from build123d import *

# Parameters (mm, degrees)
SKETCH1_W                    = 63.5
SKETCH1_H                    = 152.4
BASE_FLANGE1_DEPTH           = 1.5875
EDGE_FLANGE1_STRIP_W         = 9.525
EDGE_FLANGE1_STRIP_H         = 1.5875
EDGE_FLANGE1_STRIP_CUT_DEPTH = 152.4
EDGE_FLANGE1_DEPTH           = 152.4
EDGE_FLANGE2_STRIP_W         = 9.525
EDGE_FLANGE2_STRIP_H         = 1.5875
EDGE_FLANGE2_STRIP_CUT_DEPTH = 152.4
EDGE_FLANGE2_DEPTH           = 152.4
F_4_CLEARANCE_HOLE1_REACH    = 120.638
F_4_CLEARANCE_HOLE1_BORE_R   = 1.63195
SKETCH16_W                   = 9.525
SKETCH16_H                   = 82.55
CUT_EXTRUDE1_DEPTH           = 118.796351015


# Sheet-metal steps are written as plain solids
with BuildPart() as part:
    # Sketch1 → Base-Flange1 (new body)
    with BuildSketch(Plane.XY):
        Rectangle(SKETCH1_W, SKETCH1_H)
    extrude(amount=-BASE_FLANGE1_DEPTH)

    # Edge-Flange1 strip (across the edge) → Edge-Flange1 strip cut (cut)
    with BuildSketch(Plane(origin=(31.75, 76.2, -1.5875), x_dir=(-1, 0, 0), z_dir=(0, -1, 0))):
        with Locations((-1.5875, -0.79375)):
            Rectangle(EDGE_FLANGE1_STRIP_W, EDGE_FLANGE1_STRIP_H)
    extrude(amount=EDGE_FLANGE1_STRIP_CUT_DEPTH, mode=Mode.SUBTRACT)

    # Edge-Flange1 section (across the edge) → Edge-Flange1 (add)
    with BuildSketch(Plane(origin=(31.75, 76.2, -1.5875), x_dir=(-1, 0, 0), z_dir=(0, -1, 0))):
        with BuildLine():
            Line((0, 1.5875), (0, 31.75))
            Line((0, 31.75), (1.5875, 31.75))
            Line((1.5875, 31.75), (1.5875, 1.5875))
            ThreePointArc((1.5875, 1.5875), (2.052467985, 0.464967985), (3.175, 0))
            Line((3.175, 0), (3.175, -1.5875))
            ThreePointArc((3.175, -1.5875), (0.92993597, -0.65756403), (0, 1.5875))
        make_face()
    extrude(amount=EDGE_FLANGE1_DEPTH)

    # Edge-Flange2 strip (across the edge) → Edge-Flange2 strip cut (cut)
    with BuildSketch(Plane(origin=(-31.75, -76.2, -1.5875), x_dir=(1, 0, 0), z_dir=(0, 1, 0))):
        with Locations((-1.5875, -0.79375)):
            Rectangle(EDGE_FLANGE2_STRIP_W, EDGE_FLANGE2_STRIP_H)
    extrude(amount=EDGE_FLANGE2_STRIP_CUT_DEPTH, mode=Mode.SUBTRACT)

    # Edge-Flange2 section (across the edge) → Edge-Flange2 (add)
    with BuildSketch(Plane(origin=(-31.75, -76.2, -1.5875), x_dir=(1, 0, 0), z_dir=(0, 1, 0))):
        with BuildLine():
            Line((0, 1.5875), (0, 63.5))
            Line((0, 63.5), (1.5875, 63.5))
            Line((1.5875, 63.5), (1.5875, 1.5875))
            ThreePointArc((1.5875, 1.5875), (2.052467985, 0.464967985), (3.175, 0))
            Line((3.175, 0), (3.175, -1.5875))
            ThreePointArc((3.175, -1.5875), (0.92993597, -0.65756403), (0, 1.5875))
        make_face()
    extrude(amount=EDGE_FLANGE2_DEPTH)

    # #4 Clearance Hole1 bore → #4 Clearance Hole1 (cut, up to next)
    with BuildSketch(Plane.ZY.offset(31.75), mode=Mode.PRIVATE) as f_4_clearance_hole1_sk1:
        with Locations((-9.525, -50.8)):
            Circle(F_4_CLEARANCE_HOLE1_BORE_R)
    f_4_clearance_hole1_tool1 = extrude(f_4_clearance_hole1_sk1.sketch, amount=-F_4_CLEARANCE_HOLE1_REACH, mode=Mode.PRIVATE) & part.part
    # #4 Clearance Hole1 bore → #4 Clearance Hole1 (cut, up to next)
    with BuildSketch(Plane.ZY.offset(31.75), mode=Mode.PRIVATE) as f_4_clearance_hole1_sk2:
        with Locations((-9.525, 0)):
            Circle(F_4_CLEARANCE_HOLE1_BORE_R)
    f_4_clearance_hole1_tool2 = extrude(f_4_clearance_hole1_sk2.sketch, amount=-F_4_CLEARANCE_HOLE1_REACH, mode=Mode.PRIVATE) & part.part
    # #4 Clearance Hole1 bore → #4 Clearance Hole1 (cut, up to next)
    with BuildSketch(Plane.ZY.offset(31.75), mode=Mode.PRIVATE) as f_4_clearance_hole1_sk3:
        with Locations((-9.525, 50.8)):
            Circle(F_4_CLEARANCE_HOLE1_BORE_R)
    f_4_clearance_hole1_tool3 = extrude(f_4_clearance_hole1_sk3.sketch, amount=-F_4_CLEARANCE_HOLE1_REACH, mode=Mode.PRIVATE) & part.part
    add(f_4_clearance_hole1_tool1.solids().sort_by_distance((-31.75, -50.8, -9.525))[0], mode=Mode.SUBTRACT)
    add(f_4_clearance_hole1_tool2.solids().sort_by_distance((-31.75, 0, -9.525))[0], mode=Mode.SUBTRACT)
    add(f_4_clearance_hole1_tool3.solids().sort_by_distance((-31.75, 50.8, -9.525))[0], mode=Mode.SUBTRACT)

    # Sketch16 → Cut-Extrude1 (cut, through all)
    with BuildSketch(Plane(origin=(-30.1625, 0, 0), x_dir=(0, 0, -1), z_dir=(1, 0, 0))):
        with Locations((60.325, -4.699)):
            Rectangle(SKETCH16_W, SKETCH16_H)
    extrude(amount=-CUT_EXTRUDE1_DEPTH, mode=Mode.SUBTRACT)


solid = part.part
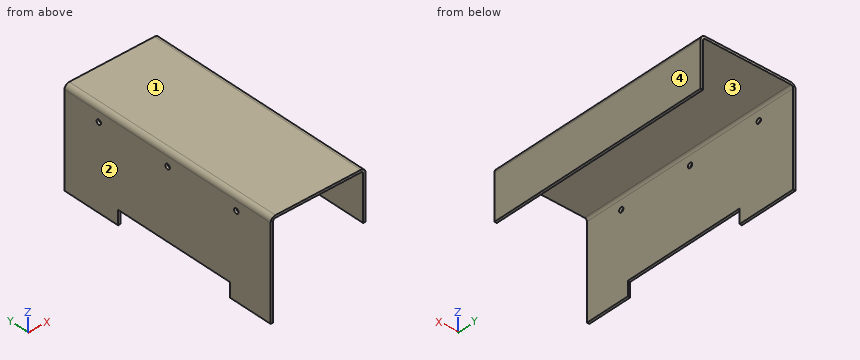
Source: CAD feature listing. Evaluate the final solid. Frame: model axes, mm. Face numbers are marked on the shaded views. Round coordinates to 2 decimals unless told otherwise and drop trailing zeros. Loops run counter-clockwise (first coordinate to the right, second up) from the corner with the lowest first, then second, coordinate; pieces in that order, holes last. Notation, with made-up numbers: M 48,32.5 L 94,32.5 A15 ccw 94,47.5 Z; hole C 41,22 d3. An arc over 180 degrees is marked long. Return JSON: item names as keys, results as strings. Group by question number.
1. Pin query (flat end, axial travel): pin 1 (5 mm diameter, centred on x = 0, y = -29.5, fed in from -Z); pin 2 (1.7 mm diameter, centred on x = 31, y = 27, fed in from -Z); pin 3 (1.3 mm diameter, centred on x = -31, y = 2.5, fed in from -Z). Return the tip coordinate at first contact, or that it passes through.
2. Section query A-A on z = -27. Output: boundary loops of the cut face in (x, y), and give its area (3 significant figures).
3. Material intervals for line 1 along X through (y, z) = (-28, -25.5); line 2 along X through (y, z) = (-48, -55); line 3 along Z through (x, y) = (5, 61.5), sorted ascending. Write a range as from..to.
4. Section query D-D on z = -60. Output: boundary loops of the cut face in (x, y), and give its area (3 significant figures).
5. Mould query, pull axis X, two halves, no side actions, for the marked faces 1, 2, 3 and 4. Classes: released by +X, released by -X, zero draft, split by the parting line, or undercut.
Checks:
{
 "1": {"pin 1": "stops at z = -1.59", "pin 2": "stops at z = -33.34", "pin 3": "stops at z = -55.56"},
 "2": {"outline": "M -31.75,-76.2 L -30.16,-76.2 L -30.16,76.2 L -31.75,76.2 Z; M 30.16,-76.2 L 31.75,-76.2 L 31.75,76.2 L 30.16,76.2 Z", "area": "484 mm²"},
 "3": {"line 1": "x = -31.75..-30.16, 30.16..31.75", "line 2": "x = -31.75..-30.16", "line 3": "z = -1.59..0"},
 "4": {"outline": "M -31.75,-76.2 L -30.16,-76.2 L -30.16,-45.97 L -31.75,-45.97 Z; M -31.75,36.58 L -30.16,36.58 L -30.16,76.2 L -31.75,76.2 Z", "area": "111 mm²"},
 "5": {"face 1": "zero draft", "face 2": "released by -X", "face 3": "undercut", "face 4": "released by +X"}
}
